Verification items for the finished model (mm, model axes). Give positions to 0.01 mm unless a question says otherwise; leave off trailing zeros. Loops run counter-clockwise (first coordinate to the right, second up) from the corner with the lowest first, then second, coordinate; pieces in that order, holes last. Notation, with made-up numbers: (32.5, -37) - (84.5, -37) arc R20 cw to (84.5, -33) - close; hole circle Ø10 at (32.5, -34.5). An arc over 180 degrees is marked (long way). One line per question, with ' | ' between items. Start each with the question number.
1. Thickness scan on line 1 along X through (y, z) = (4.8, 5.5); line 2 along Z through (x, y) = (6.5, 4.45); line 3 along X through (y, z) = (5.3, -22). Record the ranges inside material, lowest first. Write a range as from..to.
2. Section check A-A, the plane x = 6.5. Enter the section's corners in (y, z), then the cut area to 3 significant figures.
3. Depth check by flat-ended pin: pin 1 Ø3 at (x, z) = (41.43, -22.19) entering from +Y. Enter the tip coordinate at first touch or a pass-through.
4. Section check C-C, the plane y = 3.95. State how many separate pieces and enclosed holes the cut face has, then the cut area to 3 significant figures.
5. Section check B-B, the plane z = 14.5. Enter the section's corners in (x, y).
from build123d import *

# Parameters (mm, degrees)
SKETCH1_W           = 88
SKETCH1_H           = 96
BOSS_EXTRUDE1_DEPTH = 5.588
SKETCH3_R           = 1.75
CUT_EXTRUDE1_DEPTH  = 69.733665789
CUT_EXTRUDE2_DEPTH  = 69.733665789
SKETCH5_R           = 1.75
CUT_EXTRUDE3_DEPTH  = 69.733665789


with BuildPart() as part:
    # Sketch1 → Boss-Extrude1 (new body)
    with BuildSketch(Plane(origin=(0, 0, 0), x_dir=(1, 0, 0), z_dir=(0, 1, 0))):
        with Locations((1.952207024, -2.808323514)):
            Rectangle(SKETCH1_W, SKETCH1_H)
    extrude(amount=BOSS_EXTRUDE1_DEPTH)

    # Sketch3 → Cut-Extrude1 (cut, through all)
    with BuildSketch(Plane(origin=(0, 5.588, 0), x_dir=(1, 0, 0), z_dir=(0, 1, 0))):
        with Locations(Location((-24.047792976, 30.191676486, 0), (0, 0, 270))):
            Circle(SKETCH3_R)
        with Locations(Location((27.952207024, 30.191676486, 0), (0, 0, 270))):
            Circle(SKETCH3_R)
        with Locations(Location((-24.047792976, -45.708323514, 0), (0, 0, 270))):
            Circle(SKETCH3_R)
        with Locations(Location((27.952207024, -45.708323514, 0), (0, 0, 270))):
            Circle(SKETCH3_R)
        with Locations(Location((-24.547792976, 39.191676486, 0), (0, 0, 270))):
            Circle(SKETCH3_R)
        with Locations(Location((28.452207024, 39.191676486, 0), (0, 0, 270))):
            Circle(SKETCH3_R)
        with Locations(Location((-24.547792976, 10.191676486, 0), (0, 0, 270))):
            Circle(SKETCH3_R)
        with Locations(Location((28.452207024, 10.191676486, 0), (0, 0, 270))):
            Circle(SKETCH3_R)
    extrude(amount=-CUT_EXTRUDE1_DEPTH, mode=Mode.SUBTRACT)

    # Sketch4 → Cut-Extrude2 (cut, through all)
    with BuildSketch(Plane(origin=(0, 5.588, 0), x_dir=(1, 0, 0), z_dir=(0, 1, 0))):
        with BuildLine():
            Line((-9.047792976, 34.691676486), (12.952207024, 34.691676486))
            ThreePointArc((12.952207024, 34.691676486), (15.780634149, 33.52010361), (16.952207024, 30.691676486))
            Line((16.952207024, 30.691676486), (16.952207024, -36.308323514))
            ThreePointArc((16.952207024, -36.308323514), (15.780634149, -39.136750639), (12.952207024, -40.308323514))
            Line((12.952207024, -40.308323514), (-9.047792976, -40.308323514))
            ThreePointArc((-9.047792976, -40.308323514), (-11.8762201, -39.136750639), (-13.047792976, -36.308323514))
            Line((-13.047792976, -36.308323514), (-13.047792976, 30.691676486))
            ThreePointArc((-13.047792976, 30.691676486), (-11.8762201, 33.52010361), (-9.047792976, 34.691676486))
        make_face()
    extrude(amount=-CUT_EXTRUDE2_DEPTH, mode=Mode.SUBTRACT)

    # Sketch5 → Cut-Extrude3 (cut, through all)
    with BuildSketch(Plane(origin=(0, 5.588, 0), x_dir=(1, 0, 0), z_dir=(0, 1, 0))):
        with Locations(Location((-37.527792976, 32.191676486, 0), (0, 0, 270))):
            Circle(SKETCH5_R)
        with Locations(Location((41.432207024, 32.191676486, 0), (0, 0, 270))):
            Circle(SKETCH5_R)
        with Locations(Location((-37.527792976, 22.191676486, 0), (0, 0, 270))):
            Circle(SKETCH5_R)
        with Locations(Location((41.432207024, 22.191676486, 0), (0, 0, 270))):
            Circle(SKETCH5_R)
        with Locations(Location((-37.527792976, 12.191676486, 0), (0, 0, 270))):
            Circle(SKETCH5_R)
        with Locations(Location((41.432207024, 12.191676486, 0), (0, 0, 270))):
            Circle(SKETCH5_R)
        with Locations(Location((-37.527792976, 2.191676486, 0), (0, 0, 270))):
            Circle(SKETCH5_R)
        with Locations(Location((41.432207024, 2.191676486, 0), (0, 0, 270))):
            Circle(SKETCH5_R)
        with Locations(Location((-37.527792976, -7.808323514, 0), (0, 0, 270))):
            Circle(SKETCH5_R)
        with Locations(Location((41.432207024, -7.808323514, 0), (0, 0, 270))):
            Circle(SKETCH5_R)
        with Locations(Location((-37.527792976, -17.808323514, 0), (0, 0, 270))):
            Circle(SKETCH5_R)
        with Locations(Location((41.432207024, -17.808323514, 0), (0, 0, 270))):
            Circle(SKETCH5_R)
        with Locations(Location((-37.527792976, -27.808323514, 0), (0, 0, 270))):
            Circle(SKETCH5_R)
        with Locations(Location((41.432207024, -27.808323514, 0), (0, 0, 270))):
            Circle(SKETCH5_R)
        with Locations(Location((-37.527792976, -37.808323514, 0), (0, 0, 270))):
            Circle(SKETCH5_R)
        with Locations(Location((41.432207024, -37.808323514, 0), (0, 0, 270))):
            Circle(SKETCH5_R)
    extrude(amount=-CUT_EXTRUDE3_DEPTH, mode=Mode.SUBTRACT)


solid = part.part
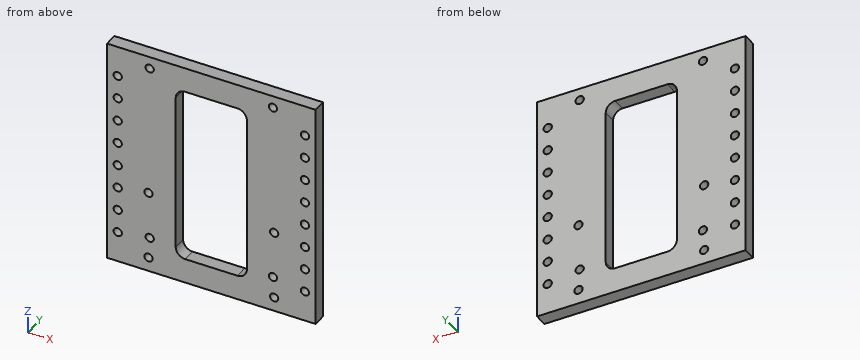
Results list:
1) line 1: -42.05..-13.05, 16.95..45.95 | line 2: -45.19..-34.69, 40.31..50.81 | line 3: -42.05..-39.27, -35.79..-13.05, 16.95..39.69, 43.17..45.95
2) outline: (0, -45.19) - (5.59, -45.19) - (5.59, -34.69) - (0, -34.69) - close; (0, 40.31) - (5.59, 40.31) - (5.59, 50.81) - (0, 50.81) - close | area: 117 mm²
3) pin 1: through
4) separate pieces: 1 | enclosed holes: 25 | area: 5,980 mm²
5) outline: (-42.05, 0) - (-13.05, 0) - (-13.05, 5.59) - (-42.05, 5.59) - close; (16.95, 0) - (45.95, 0) - (45.95, 5.59) - (16.95, 5.59) - close
